```python
from build123d import *

# Parameters (mm, degrees)
SKETCH1_R           = 5.95
SKETCH1_R_2         = 3.1
BOSS_EXTRUDE1_DEPTH = 0.4
BOSS_EXTRUDE2_START = 2
SKETCH2_R           = 3.1
BOSS_EXTRUDE2_DEPTH = 2


with BuildPart() as part:
    # Sketch1 → Boss-Extrude1 (new body)
    with BuildSketch(Plane(origin=(0, 0, 0), x_dir=(1, 0, 0), z_dir=(0, 1, 0))):
        with Locations(Location((0, 0, 0), (0, 0, 270))):
            Circle(SKETCH1_R)
        with Locations(Location((0, 0, 0), (0, 0, 270))):
            Circle(SKETCH1_R_2, mode=Mode.SUBTRACT)
    extrude(amount=-BOSS_EXTRUDE1_DEPTH)

    # Sketch2 → Boss-Extrude2 (add)
    with BuildSketch(Plane(origin=(0, 0, 0), x_dir=(1, 0, 0), z_dir=(0, 1, 0)).offset(BOSS_EXTRUDE2_START)):
        Polygon((-4, -2.309401077), (0, -4.618802154), (4, -2.309401077), (4, 2.309401077), (0, 4.618802154), (-4, 2.309401077), align=None)
        with Locations(Location((0, 0, 0), (0, 0, 270))):
            Circle(SKETCH2_R, mode=Mode.SUBTRACT)
    extrude(amount=-BOSS_EXTRUDE2_DEPTH)


solid = part.part
```
The listing builds one solid part. Answer for the finished solid, in the listing's coordinates (mm). A direction names the side the tool comes from. Coordinates: 2 decimals unless noted, no trailing zeros. Write each loop counter-clockwise with the first axis right and the second up, starting at its lowest first coordinate (ties: lowest second). Pieces come first, ordered by that corner, then holes.
Q1. Find the intervals of material crossed by line 1 along X through (y, z) = (1.05, 0); line 2 along Z through (x, y) = (1.25, 1.75); line 3 along Z through (x, y) = (-2.75, 0.4), in increasing order.
Returned:
line 1: x = -4 to -3.1, 3.1 to 4
line 2: z = -3.9 to -2.84, 2.84 to 3.9
line 3: z = -3.03 to -1.43, 1.43 to 3.03
Q2. Section D-D, the plane x = 5 is taken. Write down the section's boundary in (y, z), then the cut area to 3 significant figures.
Returned:
outline: (-0.4, -3.23) - (0, -3.23) - (0, 3.23) - (-0.4, 3.23) - close
area: 2.58 mm2
Q3. The mould has two halves that part along Z. Classify faces 1 (the cylindrical face through (0.931, 0.817, 2.957)), 2 (the flat face through (2.028, 1.014, -3.448)), 3 (the flat face through (1.4, 0, -4)): released by +Z, released by -Z, zero draft, split by the parting line, or undercut.
Returned:
face 1: undercut
face 2: released by -Z
face 3: zero draft
Q4. Section B-B, the plane x = -2.5 is taken. Write down the section's boundary in (y, z), then the cut area to 3 significant figures.
Returned:
outline: (-0.4, -5.4) - (0, -5.4) - (0, -3.18) - (2, -3.18) - (2, -1.83) - (-0.4, -1.83) - close; (-0.4, 1.83) - (2, 1.83) - (2, 3.18) - (0, 3.18) - (0, 5.4) - (-0.4, 5.4) - close
area: 8.22 mm2
Q5. Section C-C, the plane y = 0.9 is taken. Write down the section's boundary in (x, z).
Returned:
outline: (-4, -2.31) - (0, -4.62) - (4, -2.31) - (4, 2.31) - (0, 4.62) - (-4, 2.31) - close; hole circle Ø6.2 at (0, 0)
Q6. Given P1, Ø1, axis at y = 1.5, z = -4, coming from the -X side; P2, Ø6, axis at x = -0.5, z = -0.5, coming from the +Y side; P3, Ø0.6, axis at y = 0.5, z = 0.5, coming from the +X side; P4, Ø5, axis at x = 0, z = 0, coming from the -Y side, each flat-ended and moving along its own axis, determine where each tip first touches the part or whether it passes through.
Returned:
P1: stops at x = -1.94
P2: stops at y = 2
P3: stops at x = 4
P4: passes through
Q7. Which of the six approach directions +Z, -Z, +X, -X, +Y, -Y give full straight-line access (tool end or side, diameter ignored) to faces 4 (the flat face through (-1.97, 1.01, -3.48)), 5 (the flat face through (-4, 1, 0)), 6 (the flat face through (4, 1, 0))?
Returned:
face 4: -Z, -X, +Y
face 5: +Z, -Z, -X, +Y
face 6: +Z, -Z, +X, +Y
Q8. Section A-A, the plane z = 0 is taken. Write down the section's boundary in (x, y), then the cut area to 3 significant figures.
Returned:
outline: (-5.95, -0.4) - (-3.1, -0.4) - (-3.1, 2) - (-4, 2) - (-4, 0) - (-5.95, 0) - close; (3.1, -0.4) - (5.95, -0.4) - (5.95, 0) - (4, 0) - (4, 2) - (3.1, 2) - close
area: 5.88 mm2
